Can you work these out from the drawing? Everything is in mm from the part's minimum corner. A direction names the side the tool comes from. Round coordinates to 2 decimals unless told otherwise and drop trailing zeros. Write each loop counter-clockwise with the first axis right and the second up, starting at its lowest first coordinate (ties: lowest second). Pieces come first, ordered by that corner, then holes.
Q1. For the marked faces 4, 5 and 6, which set-ups out of +Z, -Z, +X, -X, +Y, -Y let a thin tool reach every point of the face, with its end or its side?
Q2. If we section it at B-B (y = 38): Please give me the cut outline in (x, z), plus the area to 3 significant figures.
Q3. If we section it at D-D (z = 23.5): Please give me the cut outline in (x, y).
Q4. I'm going to push flat-ended pins straight in: pin 1 Ø6 at (x, z) = (47.5, 39.5) entering from -Y; pin 2 Ø6 at (x, z) = (90, 37.5) entering from -Y; pin 3 Ø13 at (x, z) = (90, 12.5) entering from -Y; pin 4 Ø4 at (y, z) = (8, 17) entering from -X. Where does each tip first touch, or does it pass through?
Q5. If we section it at C-C (x = 10): Please give me the cut outline in (y, z), plus the area to 3 significant figures.
Q6. Please list where these lines run through material, in increasing order: line 1 along Z through (x, y) = (10, 43.3); line 2 along X through (y, z) = (30, 6); line 3 along X through (y, z) = (41, 37).
Q7. We'd pull the mould along X, two halves only. Please class the marked faces 1, 2 and 3: +X half, -X half, draft (parallel to the pull), parting line (faces both ways), or undercut.
Q8. If we section it at A-A (z = 37.5): Please give me the cut outline in (x, y), plus the area to 3 significant figures.
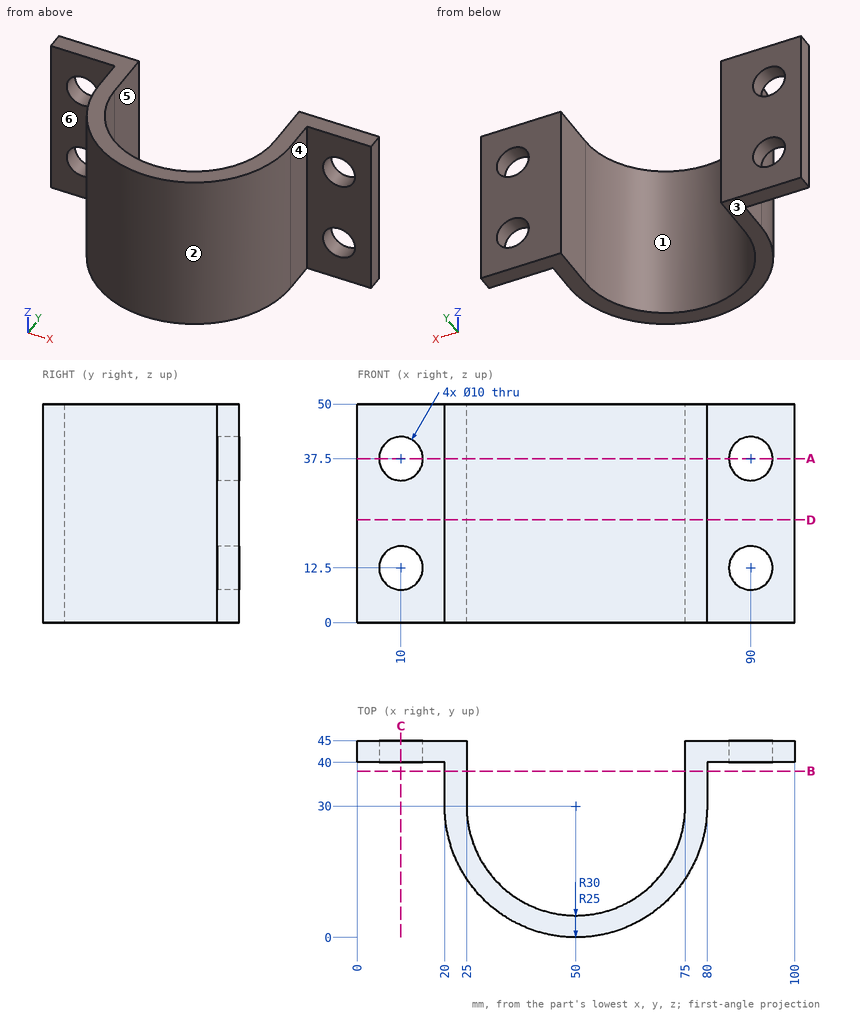
A:
1. face 4: +Z, -Z, +X, -Y
1. face 5: +Z, -Z, +Y
1. face 6: +Z, -Z, -X, -Y
2. outline: (20, 0) - (25, 0) - (25, 50) - (20, 50) - close; (75, 0) - (80, 0) - (80, 50) - (75, 50) - close
2. area: 500 mm2
3. outline: (0, 40) - (20, 40) - (20, 30) arc R30 ccw to (80, 30) - (80, 40) - (100, 40) - (100, 45) - (75, 45) - (75, 30) arc R25 cw to (25, 30) - (25, 45) - (0, 45) - close
4. pin 1: stops at y = 0
4. pin 2: passes through
4. pin 3: stops at y = 40
4. pin 4: stops at x = 27.64
5. outline: (40, 0) - (45, 0) - (45, 7.5) - (40, 7.5) - close; (40, 17.5) - (45, 17.5) - (45, 32.5) - (40, 32.5) - close; (40, 42.5) - (45, 42.5) - (45, 50) - (40, 50) - close
5. area: 150 mm2
6. line 1: z = 0 to 7.5, 17.5 to 32.5, 42.5 to 50
6. line 2: x = 20 to 25, 75 to 80
6. line 3: x = 0 to 5.03, 14.97 to 25, 75 to 85.03, 94.97 to 100
7. face 1: undercut
7. face 2: parting line
7. face 3: draft
8. outline: (0, 40) - (5, 40) - (5, 45) - (0, 45) - close; (15, 40) - (20, 40) - (20, 30) arc R30 ccw to (80, 30) - (80, 40) - (85, 40) - (85, 45) - (75, 45) - (75, 30) arc R25 cw to (25, 30) - (25, 45) - (15, 45) - close; (95, 40) - (100, 40) - (100, 45) - (95, 45) - close
8. area: 682 mm2
